```python
from build123d import *

# Parameters (mm, degrees)
SKETCH2_W           = 136
SKETCH2_H           = 92
BOSS_EXTRUDE1_DEPTH = 12
CUT_EXTRUDE1_DEPTH  = 12


with BuildPart() as part:
    # Sketch2 → Boss-Extrude1 (new body)
    with BuildSketch(Plane(origin=(0, 0, 0), x_dir=(1, 0, 0), z_dir=(0, 1, 0))):
        with Locations((68, 46)):
            Rectangle(SKETCH2_W, SKETCH2_H)
    extrude(amount=BOSS_EXTRUDE1_DEPTH)

    # Sketch2<3> → Cut-Extrude1 (cut)
    with BuildSketch(Plane(origin=(0, 0, 0), x_dir=(1, 0, 0), z_dir=(0, 1, 0))):
        with BuildLine():
            Line((23, 61), (113, 61))
            ThreePointArc((113, 61), (128, 46), (113, 31))
            Line((113, 31), (23, 31))
            ThreePointArc((23, 31), (8, 46), (23, 61))
        make_face()
    extrude(amount=CUT_EXTRUDE1_DEPTH, mode=Mode.SUBTRACT)


solid = part.part
```
Input: part model. Units: mm. Frame: model coordinates. A direction names the side the tool comes from. Round coordinates to 2 decimals unless told otherwise and drop trailing zeros. Loops run counter-clockwise (first coordinate to the right, second up) from the corner with the lowest first, then second, coordinate; pieces in that order, holes last. Notation, with made-up numbers: (-23.5, 79.25) - (0.5, 79.25) arc R19 cw to (0.5, 85.25) - close; hole circle Ø8 at (75, -26). An arc over 180 degrees is marked (long way). One line per item, written item: value. Start each with the question number.
(1) Section B-B, the plane x = 33. Return loops of the section in (y, z), plus the area to 3 significant figures.
(2) Contact query for a flat-ended pin moving along its axis: P1, Ø5, axis at x = 110.5, z = -17, coming from the -Y side. Output: stop coordinate, or through.
(3) Section C-C, the plane y = 4.5. Return loops of the section in (x, z), plus the area to 3 significant figures.
(4) Access query for faces 4 (the flat face through (67, 6, 0)), 5 (the cylindrical face through (128, 6, -46)). Directions: +Z, -Z, +X, -X, +Y, -Y. A direction counts if a zero-diameter tool reaches every point of the face in a straight line with its end or side. Return the directions, or none.
(5) Ray query, line 1 (Z direction, x = 87.5, y = 2.25); line 2 (Z direction, x = 16.5, y = 1). Return the intervals inside material, ascending. Write a range as [from, to].
(6) Section A-A, the plane z = -46. Return loops of the section in (x, y), plus the area to 3 significant figures.
(7) Draft query along X for faces 1 (the flat face through (0, 6, -45)), 2 (the cylindrical face through (8, 6, -46)), 3 (the flat face through (67, 0, -26)). Return one class per face: +X half, -X half, draft (parallel to the pull), parting line (faces both ways), or undercut.
Results below:
1. outline: (0, -92) - (12, -92) - (12, -61) - (0, -61) - close; (0, -31) - (12, -31) - (12, 0) - (0, 0) - close
1. area: 744 mm^2
2. P1: y = 0
3. outline: (0, -92) - (136, -92) - (136, 0) - (0, 0) - close; hole (23, -61) - (113, -61) arc R15 ccw to (113, -31) - (23, -31) arc R15 ccw to start
3. area: 9,110 mm^2
4. face 4: +Z, +X, -X, +Y, -Y
4. face 5: +Y, -Y
5. line 1: [-92, -61], [-31, 0]
5. line 2: [-92, -59.52], [-32.48, 0]
6. outline: (0, 0) - (8, 0) - (8, 12) - (0, 12) - close; (128, 0) - (136, 0) - (136, 12) - (128, 12) - close
6. area: 192 mm^2
7. face 1: -X half
7. face 2: undercut
7. face 3: draft
